Check sheet for the modelled part. Datum: model origin and axes. Units: mm. Round coordinates to 2 decimals unless told otherwise and drop trailing zeros. Write each loop counter-clockwise with the first axis right and the second up, starting at its lowest first coordinate (ties: lowest second). Pieces come first, ordered by that corner, then holes. Notation, with made-up numbers: (77, 40.25) -> (95, 40.25) arc R25 cw to (95, 67.25) -> close; hole circle Ø2 at (41, 65). An arc over 180 degrees is marked (long way). One line per item, written item: value.
from build123d import *

# Parameters (mm, degrees)
F2_R     = 7.5
F2_R_2   = 5.5
F3_DEPTH = 3
F4_DEPTH = 5


# Not quite as in the source:
# - a feature names something its author has since deleted; it is built from what else it names


with BuildPart() as f3:
    # F2 (on Top) → F3 (new body)
    with BuildSketch(Plane.XY):
        with BuildLine():
            Line((180, 9.5), (0, 9.5))
            ThreePointArc((0, 9.5), (-6.7175144213, 6.7175144213), (-9.5, 0))
            ThreePointArc((-9.5, 0), (-6.7175144213, -6.7175144213), (0, -9.5))
            Line((0, -9.5), (180, -9.5))
            ThreePointArc((180, -9.5), (186.7175144213, -6.7175144213), (189.5, 0))
            ThreePointArc((189.5, 0), (186.7175144213, 6.7175144213), (180, 9.5))
        make_face()
        Circle(F2_R, mode=Mode.SUBTRACT)
        with Locations((20, 0)):
            Circle(F2_R, mode=Mode.SUBTRACT)
        with Locations((40, 0)):
            Circle(F2_R, mode=Mode.SUBTRACT)
        with Locations((60, 0)):
            Circle(F2_R, mode=Mode.SUBTRACT)
        with Locations((80, 0)):
            Circle(F2_R, mode=Mode.SUBTRACT)
        with Locations((100, 0)):
            Circle(F2_R, mode=Mode.SUBTRACT)
        with Locations((120, 0)):
            Circle(F2_R, mode=Mode.SUBTRACT)
        with Locations((140, 0)):
            Circle(F2_R, mode=Mode.SUBTRACT)
        with Locations((160, 0)):
            Circle(F2_R, mode=Mode.SUBTRACT)
        with Locations((180, 0)):
            Circle(F2_R, mode=Mode.SUBTRACT)
        Circle(F2_R)
        Circle(F2_R_2, mode=Mode.SUBTRACT)
        with Locations((20, 0)):
            Circle(F2_R)
        with Locations((20, 0)):
            Circle(F2_R_2, mode=Mode.SUBTRACT)
        with Locations((40, 0)):
            Circle(F2_R)
        with Locations((40, 0)):
            Circle(F2_R_2, mode=Mode.SUBTRACT)
        with Locations((60, 0)):
            Circle(F2_R)
        with Locations((60, 0)):
            Circle(F2_R_2, mode=Mode.SUBTRACT)
        with Locations((80, 0)):
            Circle(F2_R)
        with Locations((80, 0)):
            Circle(F2_R_2, mode=Mode.SUBTRACT)
        with Locations((100, 0)):
            Circle(F2_R)
        with Locations((100, 0)):
            Circle(F2_R_2, mode=Mode.SUBTRACT)
        with Locations((120, 0)):
            Circle(F2_R)
        with Locations((120, 0)):
            Circle(F2_R_2, mode=Mode.SUBTRACT)
        with Locations((140, 0)):
            Circle(F2_R)
        with Locations((140, 0)):
            Circle(F2_R_2, mode=Mode.SUBTRACT)
        with Locations((160, 0)):
            Circle(F2_R)
        with Locations((160, 0)):
            Circle(F2_R_2, mode=Mode.SUBTRACT)
        with Locations((180, 0)):
            Circle(F2_R)
        with Locations((180, 0)):
            Circle(F2_R_2, mode=Mode.SUBTRACT)
    extrude(amount=F3_DEPTH)

    # F2 (on Top) → F4 (join)
    with BuildSketch(Plane.XY):
        Circle(F2_R)
        Circle(F2_R_2, mode=Mode.SUBTRACT)
        with Locations((20, 0)):
            Circle(F2_R)
        with Locations((20, 0)):
            Circle(F2_R_2, mode=Mode.SUBTRACT)
        with Locations((40, 0)):
            Circle(F2_R)
        with Locations((40, 0)):
            Circle(F2_R_2, mode=Mode.SUBTRACT)
        with Locations((60, 0)):
            Circle(F2_R)
        with Locations((60, 0)):
            Circle(F2_R_2, mode=Mode.SUBTRACT)
        with Locations((80, 0)):
            Circle(F2_R)
        with Locations((80, 0)):
            Circle(F2_R_2, mode=Mode.SUBTRACT)
        with Locations((100, 0)):
            Circle(F2_R)
        with Locations((100, 0)):
            Circle(F2_R_2, mode=Mode.SUBTRACT)
        with Locations((120, 0)):
            Circle(F2_R)
        with Locations((120, 0)):
            Circle(F2_R_2, mode=Mode.SUBTRACT)
        with Locations((140, 0)):
            Circle(F2_R)
        with Locations((140, 0)):
            Circle(F2_R_2, mode=Mode.SUBTRACT)
        with Locations((160, 0)):
            Circle(F2_R)
        with Locations((160, 0)):
            Circle(F2_R_2, mode=Mode.SUBTRACT)
        with Locations((180, 0)):
            Circle(F2_R)
        with Locations((180, 0)):
            Circle(F2_R_2, mode=Mode.SUBTRACT)
    extrude(amount=F4_DEPTH)


solid = f3.part
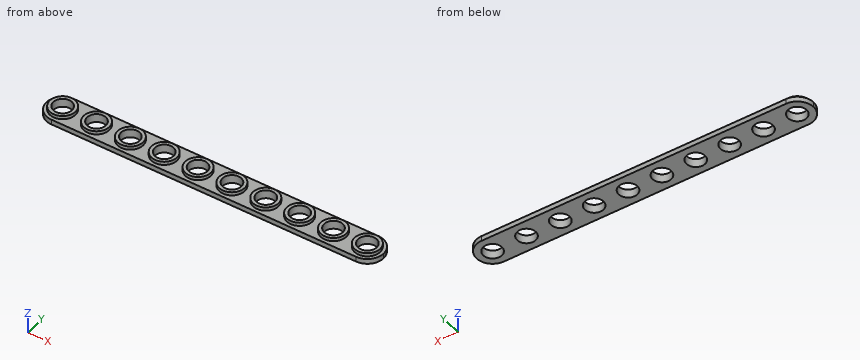
Item 1: Sectioned sample at D-D on x = 89.5. Enter the section's corners in (y, z), and give its area (3 significant figures).
Answer:
outline: (-9.5, 0) -> (9.5, 0) -> (9.5, 3) -> (-9.5, 3) -> close
area: 57.0 mm^2
Item 2: Sectioned sample at B-B on x = 160. Enter the section's corners in (y, z).
Answer:
outline: (-9.5, 0) -> (-5.5, 0) -> (-5.5, 5) -> (-7.5, 5) -> (-7.5, 3) -> (-9.5, 3) -> close; (5.5, 0) -> (9.5, 0) -> (9.5, 3) -> (7.5, 3) -> (7.5, 5) -> (5.5, 5) -> close
Item 3: Thickness scan on line 1 (Y direction, x = 180, z = 1.95); line 2 (Z direction, x = 15.5, y = -6.75); line 3 (Y direction, x = 0, z = 3.2). Record the ranges inside material, lowest first.
Answer:
line 1: y = -9.5 to -5.5, 5.5 to 9.5
line 2: z = 0 to 3
line 3: y = -7.5 to -5.5, 5.5 to 7.5
Item 4: Depth check by flat-ended pin: P1, Ø3, axis at x = 75.5, z = 3.5, coming from the -Y side; P2, Ø1.5, axis at y = -5, z = 2.5, coming from the +X side. Enter the tip coordinate at first touch or a pass-through.
Answer:
P1: stops at y = -9.5
P2: stops at x = 188.5
Item 5: Sectioned sample at A-A on z = 2.15. Count the separate pieces of the cut face and the enclosed holes in it, and give its area (3 significant figures).
Answer:
separate pieces: 1
enclosed holes: 10
area: 2,750 mm^2
